Input: part model. Units: mm. Frame: model coordinates. Coordinates: 2 decimals unless noted, no trailing zeros. Write each loop counter-clockwise with the first axis right and the second up, starting at its lowest first coordinate (ties: lowest second). Pieces come first, ordered by that corner, then holes. Notation, with made-up numbers: (59, 25) - (116, 25) arc R16 cw to (116, 46) - close; hole circle Ø11 at (59.5, 85). An arc over 180 degrees is marked (long way). Use a Markdown table: item, result. Add a question column.
Q1. Section query A-A (y = 0). Return the cut outline in (x, z).
Q2. Pin query (flat end, axial travel): P1, Ø0.8, axis at x = 9, z = 58.5, coming from the +Y side; P2, Ø5, axis at x = 0, z = 59.5, coming from the +Y side; P3, Ø1.2, axis at x = -1, z = 75, coming from the +Y side. Return the tip coordinate at first contact, or that it passes through.
Q3. Material intervals for probe 1 along Y at (x, z) = (8.25, 16); probe 2 along X at (y, z) = (7.25, 106), sorted ascending. Write a range as from..to.
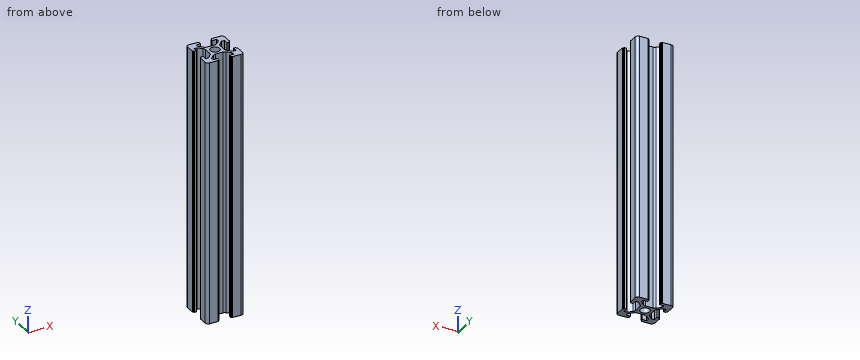
from build123d import *

# Parameters (mm, degrees)
SKETCH1_R           = 2.5
BOSS_EXTRUDE1_DEPTH = 140


with BuildPart() as part:
    # Sketch1 → Boss-Extrude1 (new body)
    with BuildSketch(Plane.XY):
        with BuildLine():
            Line((-8.5, 10), (-3.85, 10))
            ThreePointArc((-3.85, 10), (-3.673223305, 9.926776695), (-3.6, 9.75))
            Line((-3.6, 9.75), (-3.6, 9.5))
            Line((-3.6, 9.5), (-3.35, 9.5))
            ThreePointArc((-3.35, 9.5), (-3.173223305, 9.426776695), (-3.1, 9.25))
            Line((-3.1, 9.25), (-3.1, 8.2))
            Line((-3.1, 8.2), (-5.5, 8.2))
            Line((-5.5, 8.2), (-5.5, 6.560660172))
            Line((-5.5, 6.560660172), (-3.425126266, 4.485786438))
            ThreePointArc((-3.425126266, 4.485786438), (-2.776279568, 4.052240935), (-2.010912703, 3.9))
            Line((-2.010912703, 3.9), (2.010912703, 3.9))
            ThreePointArc((2.010912703, 3.9), (2.776279568, 4.052240935), (3.425126266, 4.485786438))
            Line((3.425126266, 4.485786438), (5.5, 6.560660172))
            Line((5.5, 6.560660172), (5.5, 8.2))
            Line((5.5, 8.2), (3.1, 8.2))
            Line((3.1, 8.2), (3.1, 9.25))
            ThreePointArc((3.1, 9.25), (3.173223305, 9.426776695), (3.35, 9.5))
            Line((3.35, 9.5), (3.6, 9.5))
            Line((3.6, 9.5), (3.6, 9.75))
            ThreePointArc((3.6, 9.75), (3.673223305, 9.926776695), (3.85, 10))
            Line((3.85, 10), (8.5, 10))
            ThreePointArc((8.5, 10), (9.560660172, 9.560660172), (10, 8.5))
            Line((10, 8.5), (10, 3.85))
            ThreePointArc((10, 3.85), (9.926776695, 3.673223305), (9.75, 3.6))
            Line((9.75, 3.6), (9.5, 3.6))
            Line((9.5, 3.6), (9.5, 3.35))
            ThreePointArc((9.5, 3.35), (9.426776695, 3.173223305), (9.25, 3.1))
            Line((9.25, 3.1), (8.2, 3.1))
            Line((8.2, 3.1), (8.2, 5.5))
            Line((8.2, 5.5), (6.560660172, 5.5))
            Line((6.560660172, 5.5), (4.485786438, 3.425126266))
            ThreePointArc((4.485786438, 3.425126266), (4.052240935, 2.776279568), (3.9, 2.010912703))
            Line((3.9, 2.010912703), (3.9, -2.010912703))
            ThreePointArc((3.9, -2.010912703), (4.052240935, -2.776279568), (4.485786438, -3.425126266))
            Line((4.485786438, -3.425126266), (6.560660172, -5.5))
            Line((6.560660172, -5.5), (8.2, -5.5))
            Line((8.2, -5.5), (8.2, -3.1))
            Line((8.2, -3.1), (9.25, -3.1))
            ThreePointArc((9.25, -3.1), (9.426776695, -3.173223305), (9.5, -3.35))
            Line((9.5, -3.35), (9.5, -3.6))
            Line((9.5, -3.6), (9.75, -3.6))
            ThreePointArc((9.75, -3.6), (9.926776695, -3.673223305), (10, -3.85))
            Line((10, -3.85), (10, -8.5))
            ThreePointArc((10, -8.5), (9.560660172, -9.560660172), (8.5, -10))
            Line((8.5, -10), (3.85, -10))
            ThreePointArc((3.85, -10), (3.673223305, -9.926776695), (3.6, -9.75))
            Line((3.6, -9.75), (3.6, -9.5))
            Line((3.6, -9.5), (3.35, -9.5))
            ThreePointArc((3.35, -9.5), (3.173223305, -9.426776695), (3.1, -9.25))
            Line((3.1, -9.25), (3.1, -8.2))
            Line((3.1, -8.2), (5.5, -8.2))
            Line((5.5, -8.2), (5.5, -6.560660172))
            Line((5.5, -6.560660172), (3.425126266, -4.485786438))
            ThreePointArc((3.425126266, -4.485786438), (2.776279568, -4.052240935), (2.010912703, -3.9))
            Line((2.010912703, -3.9), (-2.010912703, -3.9))
            ThreePointArc((-2.010912703, -3.9), (-2.776279568, -4.052240935), (-3.425126266, -4.485786438))
            Line((-3.425126266, -4.485786438), (-5.5, -6.560660172))
            Line((-5.5, -6.560660172), (-5.5, -8.2))
            Line((-5.5, -8.2), (-3.1, -8.2))
            Line((-3.1, -8.2), (-3.1, -9.25))
            ThreePointArc((-3.1, -9.25), (-3.173223305, -9.426776695), (-3.35, -9.5))
            Line((-3.35, -9.5), (-3.6, -9.5))
            Line((-3.6, -9.5), (-3.6, -9.75))
            ThreePointArc((-3.6, -9.75), (-3.673223305, -9.926776695), (-3.85, -10))
            Line((-3.85, -10), (-8.5, -10))
            ThreePointArc((-8.5, -10), (-9.560660172, -9.560660172), (-10, -8.5))
            Line((-10, -8.5), (-10, -3.85))
            ThreePointArc((-10, -3.85), (-9.926776695, -3.673223305), (-9.75, -3.6))
            Line((-9.75, -3.6), (-9.5, -3.6))
            Line((-9.5, -3.6), (-9.5, -3.35))
            ThreePointArc((-9.5, -3.35), (-9.426776695, -3.173223305), (-9.25, -3.1))
            Line((-9.25, -3.1), (-8.2, -3.1))
            Line((-8.2, -3.1), (-8.2, -5.5))
            Line((-8.2, -5.5), (-6.560660172, -5.5))
            Line((-6.560660172, -5.5), (-4.485786438, -3.425126266))
            ThreePointArc((-4.485786438, -3.425126266), (-4.052240935, -2.776279568), (-3.9, -2.010912703))
            Line((-3.9, -2.010912703), (-3.9, 2.010912703))
            ThreePointArc((-3.9, 2.010912703), (-4.052240935, 2.776279568), (-4.485786438, 3.425126266))
            Line((-4.485786438, 3.425126266), (-6.560660172, 5.5))
            Line((-6.560660172, 5.5), (-8.2, 5.5))
            Line((-8.2, 5.5), (-8.2, 3.1))
            Line((-8.2, 3.1), (-9.25, 3.1))
            ThreePointArc((-9.25, 3.1), (-9.426776695, 3.173223305), (-9.5, 3.35))
            Line((-9.5, 3.35), (-9.5, 3.6))
            Line((-9.5, 3.6), (-9.75, 3.6))
            ThreePointArc((-9.75, 3.6), (-9.926776695, 3.673223305), (-10, 3.85))
            Line((-10, 3.85), (-10, 8.5))
            ThreePointArc((-10, 8.5), (-9.560660172, 9.560660172), (-8.5, 10))
        make_face()
        Circle(SKETCH1_R, mode=Mode.SUBTRACT)
    extrude(amount=BOSS_EXTRUDE1_DEPTH)


solid = part.part
Values follow:
| question | item | result |
|---|---|---|
| 1 | outline | (-3.9, 0) - (-2.5, 0) - (-2.5, 140) - (-3.9, 140) - close; (2.5, 0) - (3.9, 0) - (3.9, 140) - (2.5, 140) - close |
| 2 | P1 | y = 10 |
| 2 | P2 | y = 3.96 |
| 2 | P3 | y = 3.9 |
| 3 | probe 1 | -10..-3.1, 3.1..10 |
| 3 | probe 2 | -10..-5.5, 5.5..10 |
